Can you work these out from the drawing? Everything is in mm from the part's minimum corner. A direction names the side the tool comes from. Round coordinates to 2 decimals unless told otherwise and drop trailing zeros. Write each loop counter-clockwise with the first axis right and the second up, starting at its lowest first coordinate (ties: lowest second). Pieces come first, ordered by that corner, then holes. Notation, with made-up numbers: M 39.25,67 L 82.25,67 A30 ccw 82.25,91 Z; hole C 55,26.25 d10. An arc over 180 degrees is marked long. Answer in a Markdown table with one row per item. Add a question column.
(1) Suppose I cut it at A-A, the plane x = 10. Write out the boundary of the cut face in (y, z) (1 decimal).
(2) If I drill on probe 1 along Y at (x, z) = (4.5, 5.5) (1 decimal); probe 2 along X at (y, z) = (2, 3.75) (1 decimal); probe 3 along X at (y, z) = (10.75, 6.75) (1 decimal), over which ranges is the centre line in solid material (lowest first)?
(3) If we mould it in two halves opening along X, with no side actions, what happens to the marked faces 1, 2 and 3? For each: released by +X, released by -X, zero draft, split by the parting line, or undercut.
(4) I'm going to push a flat-ended pin straight in: pin 1 (5 mm diameter, centred on x = 18, z = 4, fed in from +Y). Where does the tip first touch, or does it pass through?
(5) Suppose I cut it at D-D, the plane y = 8.5. Write out the boundary of the cut face in (x, z) (1 decimal).
(6) For the marked faces 4 and 5, which set-ups out of +Z, -Z, +X, -X, +Y, -Y let a thin tool reach every point of the face, with its end or its side?
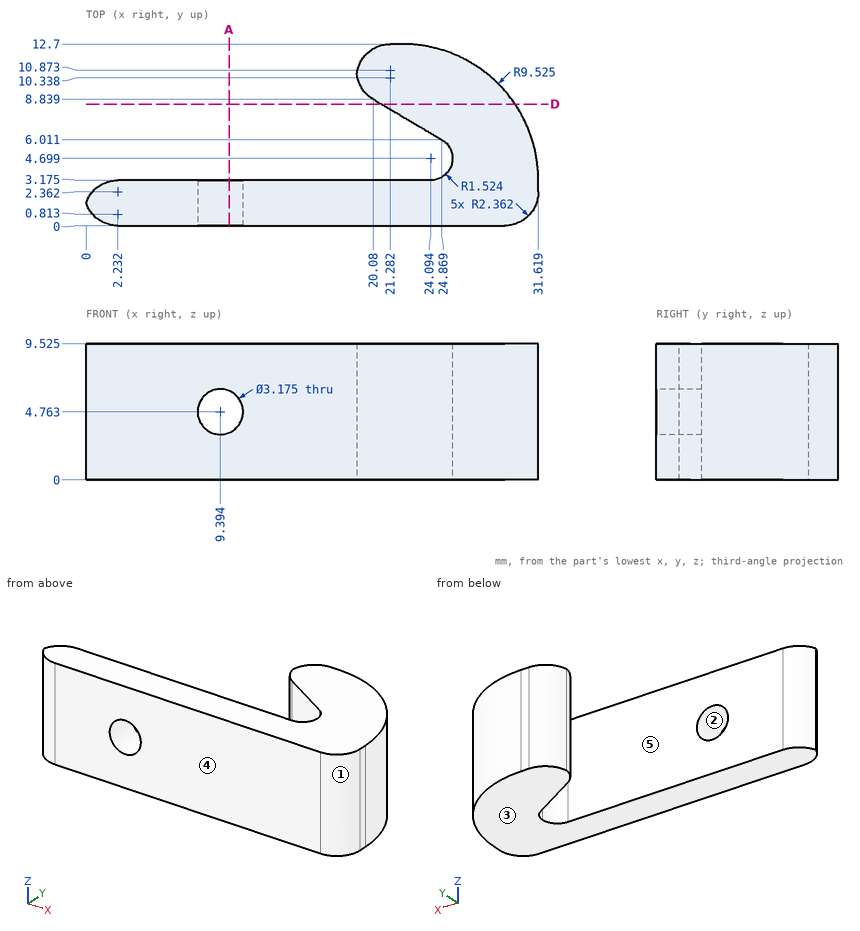
Calculated:
| question | item | result |
|---|---|---|
| 1 | outline | M 0,0 L 3.2,0 L 3.2,3.3 L 0,3.3 Z; M 0,6.2 L 3.2,6.2 L 3.2,9.5 L 0,9.5 Z |
| 2 | probe 1 | 0 to 3.2 |
| 2 | probe 2 | 0.2 to 8.2, 10.6 to 31.6 |
| 2 | probe 3 | 19 to 27.9 |
| 3 | face 1 | released by +X |
| 3 | face 2 | undercut |
| 3 | face 3 | zero draft |
| 4 | pin 1 | y = 12.57 |
| 5 | outline | M 20.7,0 L 30,0 L 30,9.5 L 20.7,9.5 Z |
| 6 | face 4 | +Z, -Z, +X, -X, -Y |
| 6 | face 5 | +Z, -Z, -X |
